from build123d import *

# Parameters (mm, degrees)
F1_DEPTH = 63.5
F2_DEPTH = 25.4
F3_DEPTH = 7.9375
F4_DEPTH = 25.4
F6_R     = 6.35


# Not quite as in the source:
# - a feature names something its author has since deleted; it is built from what else it names


with BuildPart() as f1:
    # F0 (on Front) → F1 (new body, symmetric)
    with BuildSketch(Plane.XZ):
        Polygon((-41.275, 9.525), (-41.275, -9.525), (41.275, -9.525), (41.275, 9.525), (22.225, 9.525), align=None)
    extrude(amount=F1_DEPTH, both=True)

    # F0 (on Front) → F2 (join, symmetric)
    with BuildSketch(Plane.XZ):
        with BuildLine():
            Line((22.225, 9.525), (41.275, 9.525))
            Line((41.275, 9.525), (41.275, 26.9875))
            ThreePointArc((41.275, 26.9875), (45.9246798487, 38.2128201513), (57.15, 42.8625))
            Line((57.15, 42.8625), (60.325, 42.8625))
            Line((60.325, 42.8625), (60.325, 61.9125))
            Line((60.325, 61.9125), (57.15, 61.9125))
            add(Edge.make_bspline(
                [(56.6876973993, 61.9094401137), (56.8419218796, 61.9106607794), (56.996023665, 61.9116806988), (57.15, 61.9125)],
                knots=[111.1067595469, 111.1067595469, 111.1067595469, 111.1067595469, 111.4985685166, 111.4985685166, 111.4985685166, 111.4985685166], degree=3))
            ThreePointArc((56.6876973993, 61.9094401137), (32.2913843574, 51.5192111783), (22.225, 26.9875))
            Line((22.225, 26.9875), (22.225, 9.525))
        make_face()
    extrude(amount=F2_DEPTH, both=True)

    # F0 (on Front) → F3 (join, symmetric)
    with BuildSketch(Plane.XZ):
        with BuildLine():
            add(Edge.make_bspline(
                [(-41.275, 9.525), (-40.6467419825, 45.0743155721), (12.9536750235, 61.5632913076), (56.6876973993, 61.9094401137)],
                knots=[0, 0, 0, 0, 111.1067595469, 111.1067595469, 111.1067595469, 111.1067595469], degree=3))
            Line((-41.275, 9.525), (22.225, 9.525))
            Line((22.225, 9.525), (22.225, 26.9875))
            ThreePointArc((22.225, 26.9875), (32.2913843574, 51.5192111783), (56.6876973993, 61.9094401137))
        make_face()
    extrude(amount=F3_DEPTH, both=True)

    # F0 (on Front) → F4 (join, symmetric)
    with BuildSketch(Plane.XZ):
        Polygon((81.1691840627, 61.9125), (60.325, 61.9125), (60.325, 42.8625), (81.1691840627, 42.8625), (81.1691840627, 52.7276583016), align=None)
    extrude(amount=F4_DEPTH, both=True)

    # F0 (on Front) → F5 (revolve)
    with BuildSketch(Plane.XZ):
        Polygon((81.1691840627, 66.675), (81.1691840627, 61.9125), (81.1691840627, 52.7276583016), (81.1691840627, 42.8625), (81.1691840627, 38.1), (111.125, 38.1), (111.125, 66.675), align=None)
    revolve(axis=Axis((81.1691840627, 0, 57.3200791508), (0, 0, 1)))

    # F6
    f6_edges = [f1.edges().sort_by_distance(p)[0] for p in [
        (-41.275, -63.5, 0),
        (41.275, -63.5, 0),
        (41.275, 63.5, 0),
        (-41.275, 63.5, 0),
    ]]
    fillet(f6_edges, radius=F6_R)


solid = f1.part
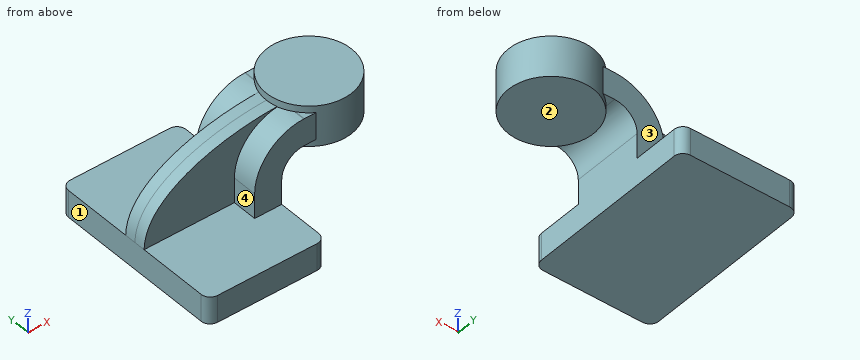
Build history of the part. All positions in model axes, mm. Face numbers are marked on the shaded views. A direction names the side the tool comes from. Round coordinates to 2 decimals unless told otherwise and drop trailing zeros. Write each loop counter-clockwise with the first axis right and the second up, starting at its lowest first coordinate (ties: lowest second). Pieces come first, ordered by that corner, then holes. Notation, with made-up numbers: M -4.75,71 L 17.25,71 A23 cw 17.25,89 Z; hole C 29.5,-4.75 d5. An arc over 180 degrees is marked long. Answer as a JSON object with one key per item and string values. Group by question number.
(1) Cut at A-A (z = 2). Give the cut face in (x, y) (3 decimals), and give its area (3 significant figures).
(2) Flat gauge pins, fed straight in: pin 1 (3.5 mm diameter, centred on x = 61, y = 21, fed in from -Z); pin 2 (2 mm diameter, centred on y = 0, z = 30.5, fed in from +X); pin 3 (6 mm diameter, centred on x = 60, y = -22, fed in from +Z) (3 decimals); pin 4 (12 mm diameter, centred on y = 33, z = 53, fed in from -X). Where does each tip first touch, or does it go through?
(3) Cut at C-C (x = 101.5). Give the cut face in (y, z) (3 decimals).
(4) Which spindle directions (+Z, -Z, +X, -X, +Y, -Y) get a long thin tool onto all of the face, cutting with end or side? Do the marked faces 1, 2, 3 and 4. Say none if no direction does.
(5) Drill centre lines: L1, parallel to Y at x = 11, z = 47; L2, parallel to Z at x = 105, y = -18 (3 decimals); L3, parallel to Z at x = -12.5, y = -39 (3 decimals). Where is each one in solid material? Low to high.
(6) Cut at B-B (y = -46.5). Give the cut face in (x, z) (3 decimals), and give its area (3 significant figures).
Responses:
{
 "1": {"outline": "M -41.275,-57.15 A6.35 ccw -34.925,-63.5 L 34.925,-63.5 A6.35 ccw 41.275,-57.15 L 41.275,57.15 A6.35 ccw 34.925,63.5 L -34.925,63.5 A6.35 ccw -41.275,57.15 Z", "area": "10,400 mm2"},
 "2": {"pin 1": "stops at z = 38.1", "pin 2": "stops at x = 41.93", "pin 3": "stops at z = 66.675", "pin 4": "stops at x = 68.19"},
 "3": {"outline": "M -22,38.1 L 22,38.1 L 22,66.675 L -22,66.675 Z"},
 "4": {"face 1": "+Z, -Z, -X, +Y, -Y", "face 2": "-Z, +X, +Y, -Y", "face 3": "+Z, -X, +Y", "face 4": "+Z, -X, -Y"},
 "5": {"L1": "y = -7.94 to 7.94", "L2": "z = 38.1 to 66.675", "L3": "z = -9.525 to 9.525"},
 "6": {"outline": "M -41.275,-9.525 L 41.275,-9.525 L 41.275,9.525 L -41.275,9.525 Z", "area": "1,570 mm2"}
}
